Print and shaded views of the part. All mm, measured from the part's lowest x, y and z. A direction names the side the tool comes from. Round coordinates to 2 decimals unless told otherwise and drop trailing zeros. Order: outer loops, then holes, each group sorted by start corner. A loop starts at its lowest first (then second) coordinate and runs counter-clockwise, first axis right, second up. Notation, with made-up numbers: (58.5, 76) - (75.5, 76) arc R20 cw to (75.5, 108) - close; hole circle Ø6 at (-18, 5.5). An arc over 180 degrees is marked (long way). Return JSON: item names as keys, results as strings. Group by question number.
Item 1: Saw through at D-D on y = 6.5. List the corners of the cut face in (x, z).
Item 2: Two-plate mould, pull along Z, no slides. Class the marked faces 4, 5 and 6: released by +Z, released by -Z, zero draft, split by the parting line, or undercut.
Item 3: Saw through at A-A on x = 69.75. List the corners of the cut face in (y, z).
Item 4: Drop flat-ended pins along their axis: pin 1 (5 mm diameter, centred on x = 68.5, z = 27.5, fed in from +Y); pin 2 (5 mm diameter, centred on x = 44.5, z = 10.5, fed in from +Y); pin 3 (4 mm diameter, centred on y = 9.5, z = 22.5, fed in from +X). Give the stop position or say it passes through.
Item 5: Saw through at B-B on z = 51.5. List the corners of the cut face in (x, y).
Item 6: Saw through at C-C on x = 7. List the corners of the cut face in (y, z), and give its area (3 significant figures).
Item 7: Probe probe 1 along Z at (x, y) = (39, 9.5); probe 2 along X at (y, z) = (9, 20.5); probe 3 along X at (y, z) = (2.25, 10.5). List the from-to ranges inside material, lowest first.
Item 8: Tool access for the marked faces 1, 2 and 3: list every direction of +Z, -Z, +X, -X, +Y, -Y with a clear straight run to the whole face (end or side of a thin tool).
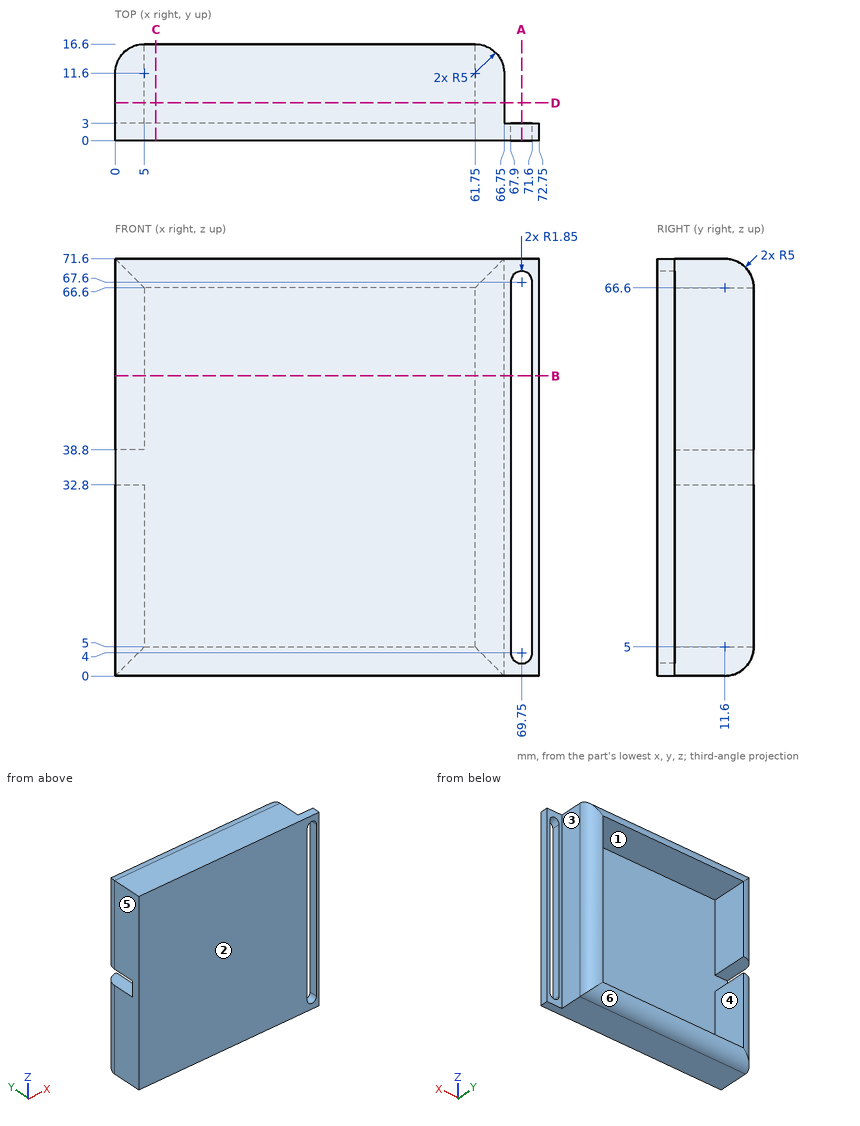
Filled in:
{
 "1": {"outline": "(0, 0) - (66.75, 0) - (66.75, 71.6) - (0, 71.6) - (0, 38.8) - (5, 38.8) - (5, 66.6) - (61.75, 66.6) - (61.75, 5) - (5, 5) - (5, 32.8) - (0, 32.8) - close"},
 "2": {"face 4": "undercut", "face 5": "zero draft", "face 6": "released by -Z"},
 "3": {"outline": "(0, 0) - (3, 0) - (3, 2.15) - (0, 2.15) - close; (0, 69.45) - (3, 69.45) - (3, 71.6) - (0, 71.6) - close"},
 "4": {"pin 1": "stops at y = 14.23", "pin 2": "stops at y = 3", "pin 3": "stops at x = 66.75"},
 "5": {"outline": "(0, 0) - (67.9, 0) - (67.9, 3) - (66.75, 3) - (66.75, 11.6) arc R5 ccw to (61.75, 16.6) - (61.75, 3) - (5, 3) - (5, 16.6) arc R5 ccw to (0, 11.6) - close; (71.6, 0) - (72.75, 0) - (72.75, 3) - (71.6, 3) - close"},
 "6": {"outline": "(0, 0) - (11.6, 0) arc R5 ccw to (16.6, 5) - (3, 5) - (3, 66.6) - (16.6, 66.6) arc R5 ccw to (11.6, 71.6) - (0, 71.6) - close", "area": "340 mm^2"},
 "7": {"probe 1": "z = 0 to 5, 66.6 to 71.6", "probe 2": "x = 0 to 5, 61.75 to 66.75", "probe 3": "x = 0 to 67.9, 71.6 to 72.75"},
 "8": {"face 1": "+Y", "face 2": "+Z, -Z, +X, -X, -Y", "face 3": "+Z, -Z, +X, +Y"}
}
